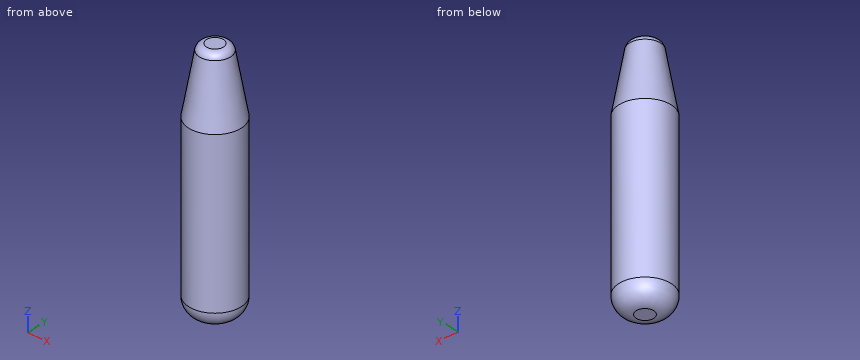
from build123d import *

# Parameters (mm, degrees)
SKETCH1_R           = 228.6
BOSS_EXTRUDE1_DEPTH = 2133.6
FILLET1_R           = 152.4
CHAMFER1_SIZE       = 101.6
CHAMFER1_SIZE2      = 576.202232873
FILLET2_R           = 63.5


with BuildPart() as part:
    # Sketch1 → Boss-Extrude1 (new body)
    with BuildSketch(Plane.XY):
        Circle(SKETCH1_R)
    extrude(amount=BOSS_EXTRUDE1_DEPTH)

    # Fillet1
    fillet1_edges = [part.edges().sort_by_distance(p)[0] for p in [
        (-228.6, 0, 0),
    ]]
    fillet(fillet1_edges, radius=FILLET1_R)

    # Chamfer1
    chamfer1_edges = [part.edges().sort_by_distance(p)[0] for p in [
        (-228.6, 0, 2133.6),
    ]]
    chamfer1_side = [part.faces().sort_by_distance(p)[0] for p in [
        (0, 0, 2133.6),
    ]]
    chamfer(chamfer1_edges, length=CHAMFER1_SIZE, length2=CHAMFER1_SIZE2, reference=chamfer1_side[0])

    # Fillet2
    fillet2_edges = [part.edges().sort_by_distance(p)[0] for p in [
        (-127, 0, 2133.6),
    ]]
    fillet(fillet2_edges, radius=FILLET2_R)


solid = part.part
Part model, mm, in its own coordinate system. Coordinates: 2 decimals unless noted, no trailing zeros. Loops run counter-clockwise (first coordinate to the right, second up) from the corner with the lowest first, then second, coordinate; pieces in that order, holes last. Notation, with made-up numbers: M 37,21.25 L 63,21.25 A15 ccw 63,42.25 Z; hole C 80.25,74.25 d3. An arc over 180 degrees is marked long. Use a Markdown table: item, result. Add a question column.
Q1. Pin check, flat tips, straight feed: P1, Ø4, axis at y = -11.5, z = 999, coming from the -X side; P2, Ø10, axis at x = 149, z = 1828.5, coming from the +Y side; P3, Ø3, axis at x = 49.5, z = 540, coming from the +Y side. Stop position of each tip, or through.
Q2. Cut at B-B (z = 1999). Write the cut outline in (x, y).
Q3. Probe L1, parallel to X at y = -8, z = 465.5; L2, parallel to Y at x = -15, z = 1433; L3, parallel to X at y = -148, z = 1289. List the from-to ranges inside material, lowest first.
Q4. Cut at A-A (z = 172). Write the cut outline in (x, y).
Worked out:
| question | item | result |
|---|---|---|
| 1 | P1 | stops at x = -228.4 |
| 1 | P2 | stops at y = 109.48 |
| 1 | P3 | stops at y = 223.5 |
| 2 | outline | C 0,0 d301.47 |
| 3 | L1 | x = -228.46 to 228.46 |
| 3 | L2 | y = -228.11 to 228.11 |
| 3 | L3 | x = -174.22 to 174.22 |
| 4 | outline | C 0,0 d457.2 |
